The listing builds one solid part. Answer for the finished solid, in the listing's coordinates (mm). A direction names the side the tool comes from. Coordinates: 2 decimals unless noted, no trailing zeros. Write each loop counter-clockwise with the first axis right and the second up, starting at its lowest first coordinate (ties: lowest second). Pieces come first, ordered by that corner, then holes.
from build123d import *

# Parameters (mm, degrees)
PAD001_DEPTH = 4.5
FILLET_R     = 3
FILLET010_R  = 12


with BuildPart() as part:
    # Sketch001 → Pad001 (new body, symmetric)
    with BuildSketch(Plane.YZ):
        with BuildLine():
            Line((-31, -31), (31, -31))
            Line((31, -31), (31, 9))
            ThreePointArc((35, 9), (33, 11), (31, 9))
            Line((35, 9), (40, 9))
            Line((40, 9), (40, 149))
            Line((40, 149), (30.6417777248, 174.7115043875))
            Line((25.9433146208, 173.0014036708), (30.6417777248, 174.7115043875))
            ThreePointArc((22.1845441377, 171.6333230975), (24.7479696659, 170.4379781426), (25.9433146208, 173.0014036708))
            Line((22.1845441377, 171.6333230975), (14.6601009845, 192.3065607548))
            Line((14.6601009845, 192.3065607548), (-39.0672095661, 172.7514189472))
            Line((-39.0672095661, 172.7514189472), (-31.5427664129, 152.0781812899))
            ThreePointArc((-35.3015368961, 150.7101007166), (-32.7381113678, 149.5147557617), (-31.5427664129, 152.0781812899))
            Line((-35.3015368961, 150.7101007166), (-40, 149))
            Line((-40, 149), (-40, 9))
            Line((-35, 9), (-40, 9))
            ThreePointArc((-31, 9), (-33, 11), (-35, 9))
            Line((-31, 9), (-31, -31))
        make_face()
        with BuildLine():
            Line((-5, 0), (5, 0))
            ThreePointArc((5, -4), (7, -2), (5, 0))
            Line((5, -4), (5, -18))
            ThreePointArc((5, -22), (7, -20), (5, -18))
            Line((5, -22), (-5, -22))
            ThreePointArc((-5, -18), (-7, -20), (-5, -22))
            Line((-5, -18), (-5, -4))
            ThreePointArc((-5, 0), (-7, -2), (-5, -4))
        make_face(mode=Mode.SUBTRACT)
        with BuildLine():
            ThreePointArc((9, 140), (0, 149), (-9, 140))
            Line((-9, 140), (-9, 36))
            ThreePointArc((-9, 36), (0, 27), (9, 36))
            Line((9, 140), (9, 36))
        make_face(mode=Mode.SUBTRACT)
    extrude(amount=PAD001_DEPTH, both=True)

    # Fillet
    fillet_edges = [part.edges().sort_by_distance(p)[0] for p in [
        (0, 30.641778, 174.711504),
        (0, -40, 149),
        (0, -40, 9),
        (0, 40, 9),
        (0, 31, -31),
        (0, -31, -31),
        (0, -39.06721, 172.751419),
        (0, 14.660101, 192.306561),
    ]]
    fillet(fillet_edges, radius=FILLET_R)

    # Fillet010
    fillet010_edges = [part.edges().sort_by_distance(p)[0] for p in [
        (0, 40, 149),
    ]]
    fillet(fillet010_edges, radius=FILLET010_R)


solid = part.part
1. Flat-ended cylindrical pins translate along their axes: P1, Ø4, axis at x = 1, z = -1.5, coming from the +Y side; P2, Ø4.5, axis at x = -1, z = -13.5, coming from the -Y side; P3, Ø1, axis at x = 2.5, z = 152, coming from the +Y side. Find the tip coordinate at first contact, or state that the pin passes through.
Results found:
P1: stops at y = 31
P2: stops at y = -31
P3: stops at y = 39.09
2. Section C-C on x = -0.75 is taken. State how many separate pieces and enclosed holes the cut face has, then the cut area to 3 significant figures.
Results found:
separate pieces: 1
enclosed holes: 2
area: 13,600 mm2
3. For a pull along Z with two mould halves and no side action, classify faces 1 (the flat face through (0.06, 18.98, 180.44)), 2 (the flat face through (0, 9, 89)), 3 (the flat face through (0, 0, -31)) as pulls with the +Z half, pulls with the -Z half, needs draft (parallel to the pull), parting line crosses it, or undercut.
Results found:
face 1: pulls with the +Z half
face 2: undercut
face 3: pulls with the -Z half
4. Find the intervals of material crossed by L1, parallel to Z at x = -3, y = 6; L2, parallel to Y at x = 3.5, z = 104; L3, parallel to Y at x = -0.75, z = -7.5, in increasing order.
Results found:
L1: z = -31 to -21.73, -18.27 to -3.73, -0.27 to 29.29, 146.71 to 189.15
L2: y = -40 to -9, 9 to 40
L3: y = -31 to -5, 5 to 31
5. Section A-A on z = 88.5 is taken. Give the vertices of the cut face in (x, y).
Results found:
outline: (-4.5, -40) - (4.5, -40) - (4.5, -9) - (-4.5, -9) - close; (-4.5, 9) - (4.5, 9) - (4.5, 40) - (-4.5, 40) - close
6. Section B-B on z = -8.5 is taken. Give the vertices of the cut face in (x, y), then the cut area to 3 significant figures.
Results found:
outline: (-4.5, -31) - (4.5, -31) - (4.5, -5) - (-4.5, -5) - close; (-4.5, 5) - (4.5, 5) - (4.5, 31) - (-4.5, 31) - close
area: 468 mm2
7. A tool of negligible diameter and unlimited length cuts with its end or side. For faces 4 (the cylindrical face through (0, -33, 11)), 5 (the flat face through (0, 31, -10)), 6 (the flat face through (0, -31, -9)), 7 (the flat face through (0, -9, 89)), 8 (the cylindrical face through (0.063, 39.823, 148.939)), from which of +Z, -Z, +X, -X, +Y, -Y can it reach the whole face along a straight path? Write none if from no direction.
Results found:
face 4: -Z, +X, -X
face 5: -Z, +X, -X, +Y
face 6: -Z, +X, -X, -Y
face 7: +X, -X
face 8: +Z, +X, -X, +Y
